Part model, mm, in its own coordinate system. Face numbers are marked on the shaded views. Coordinates: 2 decimals unless noted, no trailing zeros. Order: outer loops, then holes, each group sorted by start corner. A loop starts at its lowest first (then second) coordinate and runs counter-clockwise, first axis right, second up.
1) Wall check: L1, parallel to Y at x = 12.7, z = 7; L2, parallel to Y at x = -38.1, z = 14 (3 decimals); L3, parallel to X at y = 31.5, z = 12. Give the ranges that are in metal, low to high.
2) Cut at A-A (x = -38.1). List the corners of the cut face in (y, z) (3 decimals).
3) Cut at D-D (y = -36). List the corners of the cut face in (x, z), and give its area (3 significant figures).
4) Mould opens along Y. For the marked faces 1, 2 and 3 say: +Y half, -Y half, draft (parallel to the pull), parting line (faces both ways), or undercut.
5) Cut at C-C (x = 12.7). List the corners of the cut face in (y, z), and give its area (3 significant figures).
6) Cut at B-B (z = 14.75). List the corners of the cut face in (x, y) (3 decimals), and give its area (3 significant figures).
7) Pin check, flat tips, straight feed: pin 1 Ø8 at (x, z) = (50, 11.5) entering from -Y; pin 2 Ø8 at (x, y) = (-48, -14.5) entering from -Z. Stop position of each tip, or through.
```python
from build123d import *

# Parameters (mm, degrees)
F0_W     = 127
F0_H     = 101.6
F1_DEPTH = 19.05
F2_R     = 3.175
F3_DEPTH = 25.4
F4_R     = 6.35
F5_DEPTH = 25.4
F6_R     = 25.4


with BuildPart() as f1:
    # F0 (on Top) → F1 (new body)
    with BuildSketch(Plane.XY):
        Rectangle(F0_W, F0_H)
    extrude(amount=F1_DEPTH)

    # F2 (on face) → F3 (cut)
    with BuildSketch(Plane.XY.offset(19.05)):
        with Locations((-38.1, 25.4)):
            Circle(F2_R)
    extrude(amount=-F3_DEPTH, mode=Mode.SUBTRACT)

    # F4 (on face) → F5 (cut)
    with BuildSketch(Plane.XY.offset(19.05)):
        with Locations((12.7, -25.4)):
            Circle(F4_R)
    extrude(amount=-F5_DEPTH, mode=Mode.SUBTRACT)

    # F6
    f6_edges = [f1.edges().sort_by_distance(p)[0] for p in [
        (63.5, -50.8, 9.525),
        (63.5, 50.8, 9.525),
    ]]
    fillet(f6_edges, radius=F6_R)


solid = f1.part
```
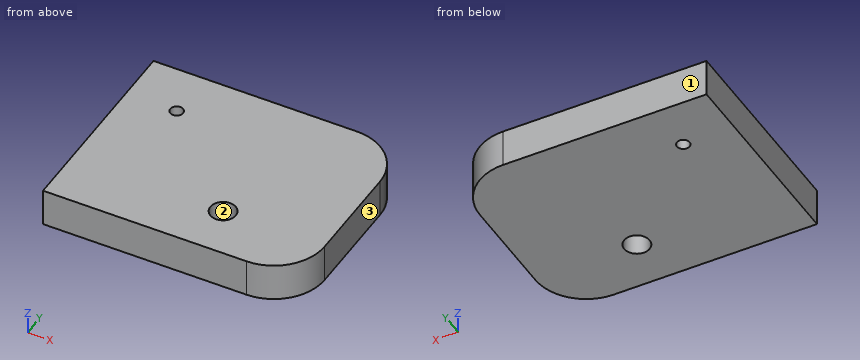
Geometry check:
1. L1: y = -50.8 to -31.75, -19.05 to 50.8
1. L2: y = -50.8 to 22.225, 28.575 to 50.8
1. L3: x = -63.5 to 62.76
2. outline: (-50.8, 0) - (22.225, 0) - (22.225, 19.05) - (-50.8, 19.05) - close; (28.575, 0) - (50.8, 0) - (50.8, 19.05) - (28.575, 19.05) - close
3. outline: (-63.5, 0) - (61.18, 0) - (61.18, 19.05) - (-63.5, 19.05) - close
3. area: 2,380 mm2
4. face 1: +Y half
4. face 2: undercut
4. face 3: draft
5. outline: (-50.8, 0) - (-31.75, 0) - (-31.75, 19.05) - (-50.8, 19.05) - close; (-19.05, 0) - (50.8, 0) - (50.8, 19.05) - (-19.05, 19.05) - close
5. area: 1,690 mm2
6. outline: (-63.5, -50.8) - (38.1, -50.8) arc R25.4 ccw to (63.5, -25.4) - (63.5, 25.4) arc R25.4 ccw to (38.1, 50.8) - (-63.5, 50.8) - close; hole circle Ø6.35 at (-38.1, 25.4); hole circle Ø12.7 at (12.7, -25.4)
6. area: 12,500 mm2
7. pin 1: stops at y = -49.54
7. pin 2: stops at z = 0
